Input: dimensioned drawing with shaded views. Units: mm. Origin: part minimum x, y, z. Round coordinates to 2 decimals unless told otherwise and drop trailing zeros. Loops run counter-clockwise (first coordinate to the right, second up) from the corner with the lowest first, then second, coordinate; pieces in that order, holes last. Notation, with made-up numbers: (28.25, 85.25) - (45.25, 85.25) arc R16 ccw to (45.25, 91.25) - close; hole circle Ø10 at (-35, -8.75). An arc over 180 degrees is marked (long way). Answer as a JSON object with one key per item and string values. Group by question number.
Item 1: Line query: line 1 (Y direction, x = 312, z = 1.75) (1 decimal); line 2 (Y direction, x = 247, z = 6). Output: solid intervals per line, ascending.
Item 2: Section A-A (x = 373). Return the cut outline in (y, z).
Item 3: Section B-B (z = 2.5). Return the cut outline in (x, y).
Item 4: First-contact query: pin 1 (1.5 mm diameter, centred on x = 183.5, z = 3, fed in from +Y) (1 decimal); pin 2 (6 mm diameter, centred on x = 287, z = 2, fed in from -Y). Flat tips, straight axial feed; report the tip coordinate or a pass-through.
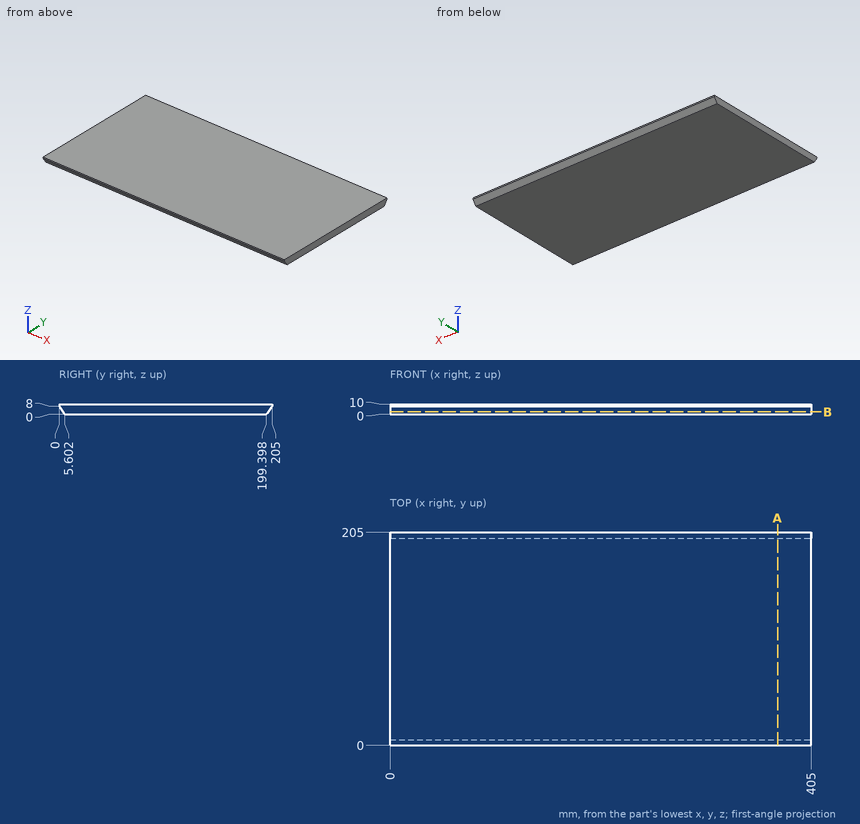
Values:
{
 "1": {"line 1": "y = 4.4 to 200.6", "line 2": "y = 1.4 to 203.6"},
 "2": {"outline": "(0, 8) - (5.6, 0) - (199.4, 0) - (205, 8) - (205, 10) - (0, 10) - close"},
 "3": {"outline": "(0, 3.85) - (405, 3.85) - (405, 201.15) - (0, 201.15) - close"},
 "4": {"pin 1": "stops at y = 202", "pin 2": "stops at y = 2.1"}
}
